from build123d import *

# Parameters (mm, degrees)
SKETCH1_R           = 1.5
BOSS_EXTRUDE1_DEPTH = 1.6


with BuildPart() as part:
    # Sketch1 → Boss-Extrude1 (new body)
    with BuildSketch(Plane(origin=(0, 0, 0), x_dir=(1, 0, 0), z_dir=(0, 1, 0))):
        Polygon((-75, -35), (-75, 35), (-45, 65), (0, 65), (0, -35), align=None)
        with Locations((-43.840620434, 43.840620434)):
            Circle(SKETCH1_R, mode=Mode.SUBTRACT)
        with Locations((-63.979633983, -15.316867676)):
            Circle(SKETCH1_R, mode=Mode.SUBTRACT)
    boss_extrude1 = extrude(amount=BOSS_EXTRUDE1_DEPTH)

    # Mirror1: Boss-Extrude1 across plane
    add(boss_extrude1.mirror(Plane(origin=(0, 1.6, 35), x_dir=(0, 0, 1), z_dir=(-1, 0, 0))))


solid = part.part
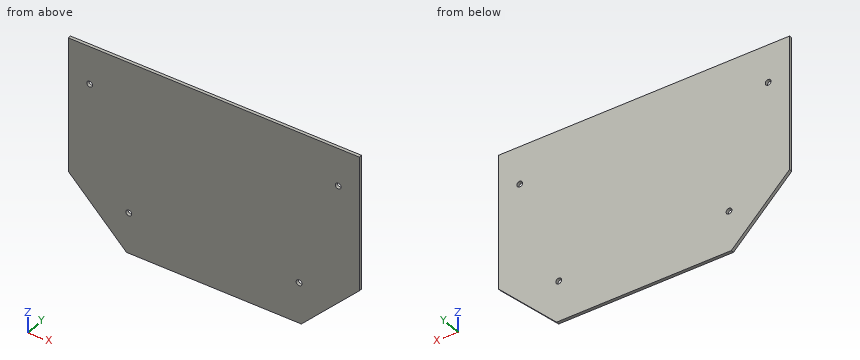
Build history of the part. All positions in model axes, mm. Round coordinates to 2 decimals unless told otherwise and drop trailing zeros. Write each loop counter-clockwise with the first axis right and the second up, starting at its lowest first coordinate (ties: lowest second). Pieces come first, ordered by that corner, then holes. Notation, with made-up numbers: M -20,2.25 L -10,2.25 A31 cw -10,27.25 Z; hole C 62.25,18.5 d5. An arc over 180 degrees is marked long. Answer in a Markdown table with one row per item.
1. Saw through at C-C (x = -55.5). List the corners of the cut face in (y, z).
Geometry check:
| item | result |
|---|---|
| outline | M 0,-54.5 L 1.6,-54.5 L 1.6,35 L 0,35 Z |
2. Probe L1, parallel to X at y = 1.35, z = -45; L2, parallel to X at y = 0.5, z = -44; L3, parallel to X at y = 1, z = -38. List the from-to ranges inside material, lowest first. Write a range as [from, to].
Geometry check:
| item | result |
|---|---|
| L1 | [-65, -44.79], [-42.89, 42.89], [44.79, 65] |
| L2 | [-66, -45.33], [-42.35, 42.35], [45.33, 66] |
| L3 | [-72, 72] |
3. Saw through at A-A (y = 1.35). List the corners of the cut face in (x, z), and give its area (3 significant figures).
Geometry check:
| item | result |
|---|---|
| outline | M -75,-35 L -45,-65 L 45,-65 L 75,-35 L 75,35 L -75,35 Z; hole C -63.98,15.32 d3; hole C -43.84,-43.84 d3; hole C 43.84,-43.84 d3; hole C 63.98,15.32 d3 |
| area | 14,100 mm2 |
4. Saw through at B-B (x = 53.5). List the corners of the cut face in (y, z).
Geometry check:
| item | result |
|---|---|
| outline | M 0,-56.5 L 1.6,-56.5 L 1.6,35 L 0,35 Z |
